```python
from build123d import *

# Parameters (mm, degrees)
F0_R     = 41.021
F1_DEPTH = 31.75
F2_R     = 34.925
F3_DEPTH = 31.751
F4_R     = 1.3589
F5_DEPTH = 44.45
F6_R     = 1.3589
F7_DEPTH = 44.45


with BuildPart() as f1:
    # F0 (on Top) → F1 (new body)
    with BuildSketch(Plane.XY):
        Circle(F0_R)
    extrude(amount=F1_DEPTH)

    # F2 (on face) → F3 (cut, through all)
    with BuildSketch(Plane.XY.offset(31.75)):
        Circle(F2_R)
    extrude(amount=-F3_DEPTH, mode=Mode.SUBTRACT)

    # F4 (on Front) → F5 (cut, symmetric)
    with BuildSketch(Plane.XZ):
        with Locations((0, 28.575)):
            Circle(F4_R)
    extrude(amount=F5_DEPTH, both=True, mode=Mode.SUBTRACT)

    # F6 (on Right) → F7 (cut, symmetric)
    with BuildSketch(Plane.YZ):
        with Locations((0, 28.575)):
            Circle(F6_R)
    extrude(amount=F7_DEPTH, both=True, mode=Mode.SUBTRACT)


solid = f1.part
```
CAD build for the part. Positions are in the model's coordinates, mm. Coordinates: 2 decimals unless noted, no trailing zeros. Order: outer loops, then holes, each group sorted by start corner. A loop starts at its lowest first (then second) coordinate and runs counter-clockwise, first axis right, second up.
(1) Saw through at D-D, the plane x = -33. Write the cut outline in (y, z).
Solution:
outline: (-24.37, 0) - (-11.43, 0) - (-11.43, 31.75) - (-24.37, 31.75) - close; (11.43, 0) - (24.37, 0) - (24.37, 31.75) - (11.43, 31.75) - close
(2) Saw through at C-C, the plane y = 15. Write the cut outline in (x, z), and give its area (3 significant figures).
Solution:
outline: (-38.18, 0) - (-31.54, 0) - (-31.54, 31.75) - (-38.18, 31.75) - close; (31.54, 0) - (38.18, 0) - (38.18, 31.75) - (31.54, 31.75) - close
area: 422 mm2
(3) Saw through at A-A, the plane x = 0. Write the cut outline in (y, z) (3 decimals), and give its area (3 significant figures).
Solution:
outline: (-41.021, 0) - (-34.925, 0) - (-34.925, 27.216) - (-41.021, 27.216) - close; (-41.021, 29.934) - (-34.925, 29.934) - (-34.925, 31.75) - (-41.021, 31.75) - close; (34.925, 0) - (41.021, 0) - (41.021, 27.216) - (34.925, 27.216) - close; (34.925, 29.934) - (41.021, 29.934) - (41.021, 31.75) - (34.925, 31.75) - close
area: 354 mm2
(4) Pin check, flat tips, straight feed: pin 1 Ø2 at (y, z) = (-10.5, 10) entering from -X; pin 2 Ø8 at (y, z) = (25, 27.5) entering from -X; pin 3 Ø1 at (y, z) = (-30.5, 8.5) entering from +X. Stop position of each tip, or through.
Solution:
pin 1: stops at x = -39.91
pin 2: stops at x = -35.24
pin 3: stops at x = 27.98
(5) Mould opens along X. For faces 1 (the face through (-8.893, -40.046, 15.653)), 2 (the face through (38, -0.18, 29.92)), 3 (the face through (-27.715, -21.251, 16.097)) say: released by +X, released by -X, zero draft, split by the parting line, or undercut.
Solution:
face 1: split by the parting line
face 2: zero draft
face 3: undercut
(6) Drill centre lines: L1, parallel to X at y = 1, z = 5; L2, parallel to Z at x = 0, y = 36.75; L3, parallel to Y at x = 0, z = 7.5 (3 decimals). Where is each one in solid material? Low to high.
Solution:
L1: x = -41.01 to -34.91, 34.91 to 41.01
L2: z = 0 to 27.22, 29.93 to 31.75
L3: y = -41.021 to -34.925, 34.925 to 41.021
